```python
from build123d import *

# Parameters (mm, degrees)
SKETCH_1_R          = 27.5
SKETCH_1_R_2        = 8.05
EXTRUDE_1_DEPTH     = 2
SKETCH_2_R          = 1.525
CUT_EXTRUDE_1_DEPTH = 2
SKETCH_3_R          = 1.525
CUT_EXTRUDE_2_DEPTH = 2


with BuildPart() as part:
    # 草图1 → 凸台-拉伸1 (new body)
    with BuildSketch(Plane.XY):
        Circle(SKETCH_1_R)
        Circle(SKETCH_1_R_2, mode=Mode.SUBTRACT)
    extrude(amount=EXTRUDE_1_DEPTH)

    # 草图2 → 切除-拉伸1 (cut)
    with BuildSketch(Plane.XY.offset(2)):
        with Locations((0, 11)):
            Circle(SKETCH_2_R)
        with Locations((9.526279442, 5.5)):
            Circle(SKETCH_2_R)
        with Locations((9.526279442, -5.5)):
            Circle(SKETCH_2_R)
        with Locations((0, -11)):
            Circle(SKETCH_2_R)
        with Locations((-9.526279442, -5.5)):
            Circle(SKETCH_2_R)
        with Locations((-9.526279442, 5.5)):
            Circle(SKETCH_2_R)
    extrude(amount=-CUT_EXTRUDE_1_DEPTH, mode=Mode.SUBTRACT)

    # 草图3 → 切除-拉伸2 (cut)
    with BuildSketch(Plane.XY.offset(2)):
        with Locations((0, 24.5)):
            Circle(SKETCH_3_R)
        with Locations((17.324116139, 17.324116139)):
            Circle(SKETCH_3_R)
        with Locations((24.5, 0)):
            Circle(SKETCH_3_R)
        with Locations((17.324116139, -17.324116139)):
            Circle(SKETCH_3_R)
        with Locations((0, -24.5)):
            Circle(SKETCH_3_R)
        with Locations((-17.324116139, -17.324116139)):
            Circle(SKETCH_3_R)
        with Locations((-24.5, 0)):
            Circle(SKETCH_3_R)
        with Locations((-17.324116139, 17.324116139)):
            Circle(SKETCH_3_R)
    extrude(amount=-CUT_EXTRUDE_2_DEPTH, mode=Mode.SUBTRACT)


solid = part.part
```
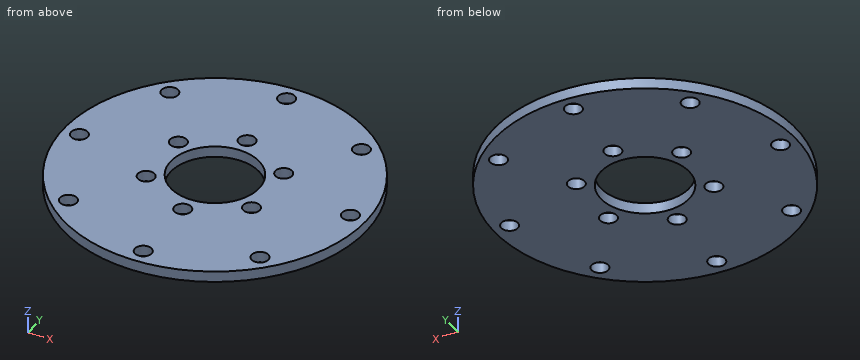
CAD build for the part. Positions are in the model's coordinates, mm. Coordinates: 2 decimals unless noted, no trailing zeros. Order: outer loops, then holes, each group sorted by start corner. A loop starts at its lowest first (then second) coordinate and runs counter-clockwise, first axis right, second up. Notation, with made-up numbers: (5, 39) -> (30, 39) arc R7 cw to (30, 50) -> close; hole circle Ø8 at (41.5, 82). An arc over 180 degrees is marked (long way). Use one line per item in the form item = value. Start each with the question number.
1) Band-saw the part on D-D on y = 0. Give the cut face in (x, z) (3 decimals).
2) Drill centre lines: L1, parallel to Y at x = 0, z = 0.85 (3 decimals); L2, parallel to Y at x = -10.5, z = 1.1; L3, parallel to Y at x = 9, z = 0.7. Where is each one in solid material? Low to high. Write a range as [from, to].
3) Band-saw the part on B-B on x = 0. Give the cut face in (y, z) (3 decimals).
4) Band-saw the part on A-A on y = 24.5. Give the cut face in (x, z) (3 decimals), then the cut area to 3 significant figures.
Entries:
q1.outline = (-27.5, 0) -> (-26.025, 0) -> (-26.025, 2) -> (-27.5, 2) -> close; (-22.975, 0) -> (-8.05, 0) -> (-8.05, 2) -> (-22.975, 2) -> close; (8.05, 0) -> (22.975, 0) -> (22.975, 2) -> (8.05, 2) -> close; (26.025, 0) -> (27.5, 0) -> (27.5, 2) -> (26.025, 2) -> close
q2.L1 = [-27.5, -26.025], [-22.975, -12.525], [-9.475, -8.05], [8.05, 9.475], [12.525, 22.975], [26.025, 27.5]
q2.L2 = [-25.42, -6.67], [-4.33, 4.33], [6.67, 25.42]
q2.L3 = [-25.99, -6.93], [-4.07, 4.07], [6.93, 25.99]
q3.outline = (-27.5, 0) -> (-26.025, 0) -> (-26.025, 2) -> (-27.5, 2) -> close; (-22.975, 0) -> (-12.525, 0) -> (-12.525, 2) -> (-22.975, 2) -> close; (-9.475, 0) -> (-8.05, 0) -> (-8.05, 2) -> (-9.475, 2) -> close; (8.05, 0) -> (9.475, 0) -> (9.475, 2) -> (8.05, 2) -> close; (12.525, 0) -> (22.975, 0) -> (22.975, 2) -> (12.525, 2) -> close; (26.025, 0) -> (27.5, 0) -> (27.5, 2) -> (26.025, 2) -> close
q4.outline = (-12.49, 0) -> (-1.525, 0) -> (-1.525, 2) -> (-12.49, 2) -> close; (1.525, 0) -> (12.49, 0) -> (12.49, 2) -> (1.525, 2) -> close
q4.area = 43.9 mm2
